from build123d import *

# Parameters (mm, degrees)
SKETCH1_W           = 25.4
SKETCH1_H           = 25.4
SKETCH1_R           = 4.7625
BOSS_EXTRUDE1_DEPTH = 12.7
SKETCH2_R           = 1.5875
CUT_EXTRUDE1_DEPTH  = 39.1


with BuildPart() as part:
    # Sketch1 → Boss-Extrude1 (new body)
    with BuildSketch(Plane(origin=(0, 0, 0), x_dir=(1, 0, 0), z_dir=(0, 1, 0))):
        with Locations((12.7, 12.7)):
            Rectangle(SKETCH1_W, SKETCH1_H)
        with Locations(Location((12.7, 12.7, 0), (0, 0, 270))):
            Circle(SKETCH1_R, mode=Mode.SUBTRACT)
    extrude(amount=BOSS_EXTRUDE1_DEPTH)

    # Sketch2 → Cut-Extrude1 (cut, through all)
    with BuildSketch(Plane.XY):
        with Locations((12.7, 6.35)):
            Circle(SKETCH2_R)
    extrude(amount=-CUT_EXTRUDE1_DEPTH, mode=Mode.SUBTRACT)


solid = part.part
Could you check a few things on this model? Use its own coordinates, in mm. Give positions to 0.01 mm unless a question says otherwise; leave off trailing zeros. Order: outer loops, then holes, each group sorted by start corner. A loop starts at its lowest first (then second) coordinate and runs counter-clockwise, first axis right, second up. Notation, with made-up numbers: (-9.5, 2) - (29.5, 2) arc R12 ccw to (29.5, 14) - close; hole circle Ø2 at (5.25, 57). An arc over 180 degrees is marked (long way). Return JSON: item names as keys, results as strings. Group by question number.
Q1. Suppose I cut it at C-C, the plane y = 6.35. Please give me the cut outline in (x, z) (1 decimal), and give its area (3 significant figures).
Q2. Please list where these lines run through material, in increasing order: line 1 along X through (y, z) = (6.35, -2.25); line 2 along Y through (x, z) = (12.7, -6); line 3 along X through (y, z) = (5.25, -12.7). Write a range as [from, to].
Q3. Suppose I cut it at A-A, the plane x = 12.7. Please give me the cut outline in (y, z).
Q4. Suppose I cut it at D-D, the plane z = -12.7. Please give me the cut outline in (x, y), and give its area (3 significant figures).
Q5. Thinking about a two-plate mould opening in Y: for faces 1 (the face through (15, 6, 0)), 2 (the face through (14.166, 5.742, -21.237)), 3 (the face through (18, 0, -13)), 4 (the face through (14.166, 5.742, -4.048)), which applies, pulls with the +Y half, pulls with the -Y half, needs draft (parallel to the pull), parting line crosses it, or undercut?
Resolved:
{
 "1": {"outline": "(0, -25.4) - (11.1, -25.4) - (11.1, -17.2) arc R4.8 cw to (11.1, -8.2) - (11.1, 0) - (0, 0) - close; (14.3, -25.4) - (25.4, -25.4) - (25.4, 0) - (14.3, 0) - (14.3, -8.2) arc R4.8 cw to (14.3, -17.2) - close", "area": "523 mm2"},
 "2": {"line 1": "x = [0, 11.11], [14.29, 25.4]", "line 2": "y = [0, 4.76], [7.94, 12.7]", "line 3": "x = [0, 7.94], [17.46, 25.4]"},
 "3": {"outline": "(0, -25.4) - (4.76, -25.4) - (4.76, -17.46) - (0, -17.46) - close; (0, -7.94) - (4.76, -7.94) - (4.76, 0) - (0, 0) - close; (7.94, -25.4) - (12.7, -25.4) - (12.7, -17.46) - (7.94, -17.46) - close; (7.94, -7.94) - (12.7, -7.94) - (12.7, 0) - (7.94, 0) - close"},
 "4": {"outline": "(0, 0) - (7.94, 0) - (7.94, 12.7) - (0, 12.7) - close; (17.46, 0) - (25.4, 0) - (25.4, 12.7) - (17.46, 12.7) - close", "area": "202 mm2"},
 "5": {"face 1": "needs draft", "face 2": "undercut", "face 3": "pulls with the -Y half", "face 4": "undercut"}
}
